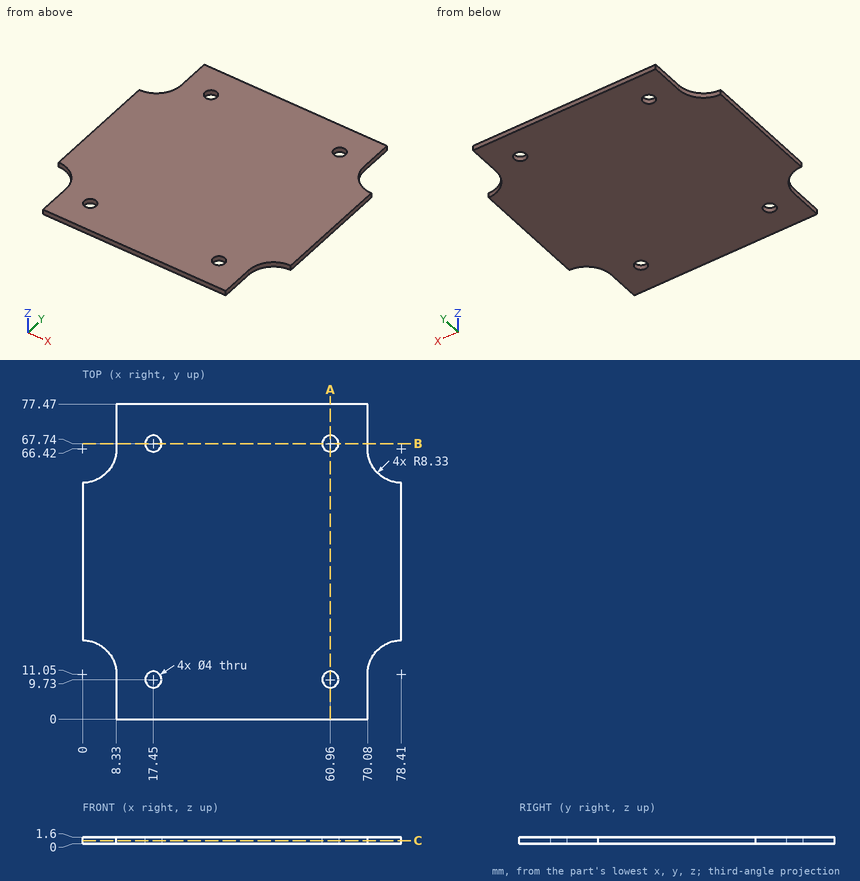
Geometry check sheet. Reference: drawing and pictorial views, mm from the part's lowest x, y, z. Coordinates: 2 decimals unless noted, no trailing zeros. Loops run counter-clockwise (first coordinate to the right, second up) from the corner with the lowest first, then second, coordinate; pieces in that order, holes last. Notation, with made-up numbers: (5.5, 79) -> (56.5, 79) arc R32 ccw to (56.5, 105) -> close; hole circle Ø8 at (83, 21.25). An arc over 180 degrees is marked (long way). Write item = value, one per line. Start each with the question number.
1. Section check C-C on z = 0.7. Record the cut outline in (x, y).
2. Section check A-A on x = 60.96. Record the cut outline in (y, z).
3. Material ranges on line 1 (Y direction, x = 17.45, z = 1.35); line 2 (X direction, y = 72.5, z = 1.2), recorded low to high.
4. Section check B-B on y = 67.74. Record the cut outline in (x, z), then the cut area to 3 significant figures.
Responses:
q1.outline = (0, 19.38) arc R8.33 cw to (8.33, 11.05) -> (8.33, 0) -> (70.08, 0) -> (70.08, 11.05) arc R8.33 cw to (78.41, 19.38) -> (78.41, 58.09) arc R8.33 cw to (70.08, 66.42) -> (70.08, 77.47) -> (8.33, 77.47) -> (8.33, 66.42) arc R8.33 cw to (0, 58.09) -> close; hole circle Ø4 at (17.45, 9.73); hole circle Ø4 at (17.45, 67.74); hole circle Ø4 at (60.96, 9.73); hole circle Ø4 at (60.96, 67.74)
q2.outline = (0, 0) -> (7.73, 0) -> (7.73, 1.6) -> (0, 1.6) -> close; (11.73, 0) -> (65.74, 0) -> (65.74, 1.6) -> (11.73, 1.6) -> close; (69.74, 0) -> (77.47, 0) -> (77.47, 1.6) -> (69.74, 1.6) -> close
q3.line_1 = 0 to 7.73, 11.73 to 65.74, 69.74 to 77.47
q3.line_2 = 8.33 to 70.08
q4.outline = (8.33, 0) -> (15.45, 0) -> (15.45, 1.6) -> (8.33, 1.6) -> close; (19.45, 0) -> (58.96, 0) -> (58.96, 1.6) -> (19.45, 1.6) -> close; (62.96, 0) -> (70.08, 0) -> (70.08, 1.6) -> (62.96, 1.6) -> close
q4.area = 86.0 mm2
